Autodesk Fusion 360 part; units mm, degrees
sketch "Sketch1" plane through (0, 0, 0) normal (0, 0, 1) x (1, 0, 0)
  line L0 (0, 0) -> (11, 0)
  line L1 (11, 0) -> (11, 22)
  line L2 (11, 22) -> (0, 22)
  line L3 (0, 22) -> (0, 0)
  line L4 (11, 0) -> (22, 0)
  line L5 (22, 0) -> (22, 11)
  line L6 (22, 11) -> (11, 11)
  line L7 (11, 11) -> (11, 0)
  dimension "d1" = 11
  dimension "d2" = 22
  dimension "d3" = 11
  dimension "d4" = 11
extrude "Extrude1" add sketch "Sketch1" along normal blind 5
sketch "Sketch2" plane through (0, 0, 5) normal (0, 0, 1) x (-1, 0, 0)
  line L0 (-22, -11) -> (-11, -11)
  line L1 (-11, -11) -> (-11, -22)
  line L2 (-11, -22) -> (0, -22)
  line L3 (0, -22) -> (0, 0)
  line L4 (0, 0) -> (-22, 0)
  line L5 (-22, 0) -> (-22, -11)
  line L6 (-22, -11) -> (-5.9353, -11)
  line L7 (-5.9353, -11) -> (-5.9353, -5.9846)
  line L8 (-5.9353, -5.9846) -> (-22, -5.9846)
  line L9 (-22, -5.9846) -> (-22, -11)
  line L10 (-5.9353, -22) -> (-11, -22)
  line L11 (-11, -22) -> (-11, -11)
  line L12 (-11, -11) -> (-5.9353, -11)
  line L13 (-5.9353, -11) -> (-5.9353, -22)
extrude "Extrude2" add sketch "Sketch2" along normal blind 3.5 contours L0 L5 L6 L7 L8 L9 L12 | L1 L2 L6 L10 L11 L12 L13
sketch "Sketch3" plane through (0, 0, 8.5) normal (0, 0, 1) x (-1, 0, 0)
  line L0 (-5.9353, -5.9846) -> (-22, -5.9846)
  line L1 (-22, -5.9846) -> (-22, -11)
  line L2 (-22, -11) -> (-11, -11)
  line L3 (-11, -11) -> (-11, -22)
  line L4 (-11, -22) -> (-5.9353, -22)
  line L5 (-5.9353, -22) -> (-5.9353, -5.9846)
  line L6 (0, -22) -> (-11, -22)
  line L7 (-11, -22) -> (-11, 0)
  line L8 (-11, 0) -> (0, 0)
  line L9 (0, 0) -> (0, -22)
  line L10 (-11, -11) -> (-22, -11)
  line L11 (-22, -11) -> (-22, 0)
  line L12 (-22, 0) -> (-11, 0)
  line L13 (-11, 0) -> (-11, -11)
extrude "Extrude3" add sketch "Sketch3" along normal blind 5
sketch "Sketch4" plane through (0, 0, 13.5) normal (0, 0, 1) x (-1, 0, 0)
  line L0 (-22, 0) -> (-22, -11)
  line L1 (-22, -11) -> (-11, -11)
  line L2 (-11, -11) -> (-11, -22)
  line L3 (-11, -22) -> (0, -22)
  line L4 (0, -22) -> (0, 0)
  line L5 (0, 0) -> (-22, 0)
  circle A0 centre (-4, -4) radius 1.5
  dimension "d11" = 3
extrude "Extrude4" cut sketch "Sketch4" against normal blind 17 contours A0
Design review of the part built by this model. Coordinates are the model's own, in mm. A direction names the side the tool comes from. Coordinates: 2 decimals unless noted, no trailing zeros. Write each loop counter-clockwise with the first axis right and the second up, starting at its lowest first coordinate (ties: lowest second). Pieces come first, ordered by that corner, then holes.
1) Mouldability with a two-part tool opening along Y and no side actions: class faces 1 (the cylindrical face through (2.57, 3.55, 2.54)), 2 (the flat face through (11, 0, 2)), 3 (the flat face through (5.935, 14, 7)) as +Y half, -Y half, draft (parallel to the pull), parting line (faces both ways), or undercut.
2) Machinability: for faces 4 (the flat face through (14, 5.985, 7)), 5 (the flat face through (9, 4, 8.5)), 6 (the flat face through (11, 16, 7)), which of the approach directions +Z, -Z, +X, -X, +Y, -Y give a long, thin tool a straight path to every point of the face, cutting with its end or side? Answer none if there is none.
3) To check wall thickness, follow L1, parallel to Z at x = 4.25, y = 18.75; L2, parallel to X at y = 4, z = 12.5. State the ranges of each line that lie inside material, in increasing order.
4) Add section A-A (y = 4). Write out the cut boundary in (x, z), plus the area to 3 significant figures.
5) Insertion check: pin 1 (3.5 mm diameter, centred on y = 19, z = 5, fed in from +X). The pin has a flat end and moves straight along its axis. Give the tip position at first contact, or say it passes through.
6) Add section C-C (z = 10.5). Write out the cut boundary in (x, y).
7) Add section D-D (x = 9). Write out the cut boundary in (y, z).
Check result:
1. face 1: undercut
1. face 2: -Y half
1. face 3: draft
2. face 4: +X, -X, -Y
2. face 5: -X, -Y
2. face 6: +Z, -Z, +X, +Y
3. L1: z = 0 to 5, 8.5 to 13.5
3. L2: x = 0 to 2.5, 5.5 to 22
4. outline: (0, 0) - (2.5, 0) - (2.5, 5) - (0, 5) - close; (0, 8.5) - (2.5, 8.5) - (2.5, 13.5) - (0, 13.5) - close; (5.5, 0) - (22, 0) - (22, 5) - (5.5, 5) - close; (5.5, 8.5) - (22, 8.5) - (22, 13.5) - (5.5, 13.5) - close
4. area: 190 mm2
5. pin 1: stops at x = 11
6. outline: (0, 0) - (22, 0) - (22, 11) - (11, 11) - (11, 22) - (0, 22) - close; hole circle Ø3 at (4, 4)
7. outline: (0, 0) - (22, 0) - (22, 13.5) - (0, 13.5) - (0, 8.5) - (5.98, 8.5) - (5.98, 5) - (0, 5) - close
